from build123d import *

# Parameters (mm, degrees)
SKETCH1_W                      = 200
SKETCH1_H                      = 120
BOSS_EXTRUDE1_DEPTH            = 100
SHELL1_T                       = -3
CUT_EXTRUDE1_REACH             = 233.517
SKETCH5_W                      = 10
SKETCH5_H                      = 10
CUT_EXTRUDE1_DIRECTION_2_DEPTH = 232.516738056
FILLET2_R                      = 10
FILLET3_R                      = 10


with BuildPart() as part:
    # Sketch1 → Boss-Extrude1 (new body)
    with BuildSketch(Plane(origin=(0, 0, 0), x_dir=(1, 0, 0), z_dir=(0, 1, 0))):
        Rectangle(SKETCH1_W, SKETCH1_H)
    extrude(amount=BOSS_EXTRUDE1_DEPTH)

    # Shell1
    shell1_openings = [part.faces().sort_by_distance(p)[0] for p in [
        (0, 100, 0),
    ]]
    offset(amount=SHELL1_T, openings=shell1_openings, kind=Kind.INTERSECTION)

    # Sketch5 → Cut-Extrude1 (cut, up to next)
    with BuildSketch(Plane(origin=(100, 0, 0), x_dir=(0, 0, -1), z_dir=(1, 0, 0)), mode=Mode.PRIVATE) as cut_extrude1_sk1:
        with Locations((-50, 10)):
            Rectangle(SKETCH5_W, SKETCH5_H)
    cut_extrude1_tool1 = extrude(cut_extrude1_sk1.sketch, amount=-CUT_EXTRUDE1_REACH, mode=Mode.PRIVATE) & part.part
    add(cut_extrude1_tool1.solids().sort_by_distance((100, 10, 50))[0], mode=Mode.SUBTRACT)

    # Sketch5 → Cut-Extrude1 direction 2 (cut)
    with BuildSketch(Plane(origin=(100, 0, 0), x_dir=(0, 0, -1), z_dir=(1, 0, 0))):
        with Locations((-50, 10)):
            Rectangle(SKETCH5_W, SKETCH5_H)
    extrude(amount=CUT_EXTRUDE1_DIRECTION_2_DEPTH, mode=Mode.SUBTRACT)

    # Fillet2
    # the kernel refuses this fillet: 10 mm, written as the material it takes off along each edge
    with BuildSketch(Plane(origin=(-100, -25, -60), x_dir=(1, 0, 0), z_dir=(0, 1, 0)), Plane(origin=(-100, -25, 60), x_dir=(0, 0, -1), z_dir=(0, 1, 0))) as fillet2_piece_1:
        with BuildLine():
            CenterArc((FILLET2_R, -FILLET2_R), FILLET2_R, 90, 90)
            Line((0, -FILLET2_R), (0, 0))
            Line((0, 0), (FILLET2_R, 0))
        make_face()
    extrude(amount=150, mode=Mode.SUBTRACT)
    with BuildSketch(Plane(origin=(100, -25, 60), x_dir=(0, 0, -1), z_dir=(0, 1, 0)), Plane(origin=(100, -25, -60), x_dir=(-1, 0, 0), z_dir=(0, 1, 0))) as fillet2_piece_2:
        with BuildLine():
            CenterArc((FILLET2_R, FILLET2_R), FILLET2_R, 180, 90)
            Line((0, FILLET2_R), (0, 0))
            Line((0, 0), (FILLET2_R, 0))
        make_face()
    extrude(amount=150, mode=Mode.SUBTRACT)

    # Fillet3
    # the kernel refuses this fillet: 10 mm, written as the material it adds along each edge
    with BuildSketch(Plane(origin=(-97, 100, 57), x_dir=(0, 0, -1), z_dir=(0, -1, 0))) as fillet3_piece_1:
        with BuildLine():
            CenterArc((FILLET3_R, FILLET3_R), FILLET3_R, 180, 90)
            Line((0, FILLET3_R), (0, 0))
            Line((0, 0), (FILLET3_R, 0))
        make_face()
    extrude(amount=97)
    with BuildSketch(Plane(origin=(97, 100, 57), x_dir=(0, 0, -1), z_dir=(0, -1, 0))) as fillet3_piece_2_section:
        with BuildLine():
            CenterArc((FILLET3_R, -FILLET3_R), FILLET3_R, 90, 90)
            Line((0, -FILLET3_R), (0, 0))
            Line((0, 0), (FILLET3_R, 0))
        make_face()
    fillet3_piece_2 = extrude(amount=97, mode=Mode.PRIVATE)
    fillet3_piece_2 = split(fillet3_piece_2, bisect_by=Plane(origin=(96.033482281, 15, 52.791302356), z_dir=(0, 1, 0)), keep=Keep.TOP, mode=Mode.PRIVATE)
    fillet3_piece_2 = split(fillet3_piece_2, bisect_by=Plane(origin=(96.033482281, 57.5, 55), z_dir=(0, 0, -1)), keep=Keep.TOP, mode=Mode.PRIVATE)
    add(fillet3_piece_2)
    with BuildSketch(Plane(origin=(97, 100, 57), x_dir=(0, 0, -1), z_dir=(0, -1, 0))) as fillet3_piece_3_section:
        with BuildLine():
            CenterArc((FILLET3_R, -FILLET3_R), FILLET3_R, 90, 90)
            Line((0, -FILLET3_R), (0, 0))
            Line((0, 0), (FILLET3_R, 0))
        make_face()
    fillet3_piece_3 = extrude(amount=97, mode=Mode.PRIVATE)
    fillet3_piece_3 = split(fillet3_piece_3, bisect_by=Plane(origin=(93.714174943, 15, 56.26775421), z_dir=(0, 1, 0)), keep=Keep.TOP, mode=Mode.PRIVATE)
    fillet3_piece_3 = split(fillet3_piece_3, bisect_by=Plane(origin=(93.714174943, 57.5, 55), z_dir=(0, 0, 1)), keep=Keep.TOP, mode=Mode.PRIVATE)
    add(fillet3_piece_3)
    with BuildSketch(Plane(origin=(97, 100, 57), x_dir=(0, 0, -1), z_dir=(0, -1, 0))) as fillet3_piece_4_section:
        with BuildLine():
            CenterArc((FILLET3_R, -FILLET3_R), FILLET3_R, 90, 90)
            Line((0, -FILLET3_R), (0, 0))
            Line((0, 0), (FILLET3_R, 0))
        make_face()
    fillet3_piece_4 = extrude(amount=97, mode=Mode.PRIVATE)
    fillet3_piece_4 = split(fillet3_piece_4, bisect_by=Plane(origin=(93.714174943, 15, 56.26775421), z_dir=(0, -1, 0)), keep=Keep.TOP, mode=Mode.PRIVATE)
    fillet3_piece_4 = split(fillet3_piece_4, bisect_by=Plane(origin=(93.714174943, 10, 55), z_dir=(0, 0, 1)), keep=Keep.TOP, mode=Mode.PRIVATE)
    fillet3_piece_4 = split(fillet3_piece_4, bisect_by=Plane(origin=(93.714174943, 5, 56.26775421), z_dir=(0, 1, 0)), keep=Keep.TOP, mode=Mode.PRIVATE)
    add(fillet3_piece_4)
    with BuildSketch(Plane(origin=(97, 100, 57), x_dir=(0, 0, -1), z_dir=(0, -1, 0))) as fillet3_piece_5_section:
        with BuildLine():
            CenterArc((FILLET3_R, -FILLET3_R), FILLET3_R, 90, 90)
            Line((0, -FILLET3_R), (0, 0))
            Line((0, 0), (FILLET3_R, 0))
        make_face()
    fillet3_piece_5 = extrude(amount=97, mode=Mode.PRIVATE)
    fillet3_piece_5 = split(fillet3_piece_5, bisect_by=Plane(origin=(96.033482281, 4, 55), z_dir=(0, 0, -1)), keep=Keep.TOP, mode=Mode.PRIVATE)
    fillet3_piece_5 = split(fillet3_piece_5, bisect_by=Plane(origin=(96.033482281, 5, 52.791302356), z_dir=(0, -1, 0)), keep=Keep.TOP, mode=Mode.PRIVATE)
    add(fillet3_piece_5)
    with BuildSketch(Plane(origin=(97, 100, 57), x_dir=(0, 0, -1), z_dir=(0, -1, 0))) as fillet3_piece_6_section:
        with BuildLine():
            CenterArc((FILLET3_R, -FILLET3_R), FILLET3_R, 90, 90)
            Line((0, -FILLET3_R), (0, 0))
            Line((0, 0), (FILLET3_R, 0))
        make_face()
    fillet3_piece_6 = extrude(amount=97, mode=Mode.PRIVATE)
    fillet3_piece_6 = split(fillet3_piece_6, bisect_by=Plane(origin=(93.714174943, 4, 55), z_dir=(0, 0, 1)), keep=Keep.TOP, mode=Mode.PRIVATE)
    fillet3_piece_6 = split(fillet3_piece_6, bisect_by=Plane(origin=(93.714174943, 5, 56.26775421), z_dir=(0, -1, 0)), keep=Keep.TOP, mode=Mode.PRIVATE)
    add(fillet3_piece_6)
    with BuildSketch(Plane(origin=(-97, 3, -57), x_dir=(1, 0, 0), z_dir=(0, 1, 0)), Plane(origin=(97, 100, -57), x_dir=(-1, 0, 0), z_dir=(0, -1, 0))) as fillet3_piece_7:
        with BuildLine():
            CenterArc((FILLET3_R, -FILLET3_R), FILLET3_R, 90, 90)
            Line((0, -FILLET3_R), (0, 0))
            Line((0, 0), (FILLET3_R, 0))
        make_face()
    extrude(amount=97)


solid = part.part
Can you work these out from the model? Positions are in its coordinate system, mm. A direction names the side the tool comes from. Give positions to 0.01 mm unless a question says otherwise; leave off trailing zeros. Order: outer loops, then holes, each group sorted by start corner. A loop starts at its lowest first (then second) coordinate and runs counter-clockwise, first axis right, second up. Notation, with made-up numbers: (48, 45.25) - (65, 45.25) arc R13 ccw to (65, 55.25) - close; hole circle Ø1 at (21.5, -19). An arc over 180 degrees is marked (long way). Write each question's results on one line, items separated by ' | '.
1) Suppose I cut it at B-B, the plane x = 25.5. Write out the boundary of the cut face in (y, z).
Final values:
outline: (0, -60) - (100, -60) - (100, -57) - (3, -57) - (3, 57) - (100, 57) - (100, 60) - (0, 60) - close
2) If we mould it in two halves opening along X, with no side actions, what happens to faces 1 (the face through (-1, 51, -57)), 2 (the face through (97.15, 49.3, -56.99)), 3 (the face through (-97.15, 49.3, 56.99)), 4 (the face through (96, 10, 55))? For each: pulls with the +X half, pulls with the -X half, needs draft (parallel to the pull), parting line crosses it, or undercut.
Final values:
face 1: undercut | face 2: pulls with the +X half | face 3: pulls with the -X half | face 4: needs draft
3) On a 3-axis mill with a long thin cutter (end or side, diameter ignored), from which of +Z, -Z, +X, -X, +Y, -Y can I reach the whole of each face in a straight line? I mean faces 5 (the face through (93.99, 52.18, -54.15)), 6 (the face through (-96.99, 49.3, -57.15)), 7 (the face through (98, 5, 51)). Say none if no direction works.
Final values:
face 5: +Y | face 6: -Z, -X, +Y, -Y | face 7: +X
4) Suppose I cut it at A-A, the plane y = 58. Write out the boundary of the cut face in (x, z).
Final values:
outline: (-100, -50) arc R10 ccw to (-90, -60) - (90, -60) arc R10 ccw to (100, -50) - (100, 50) arc R10 ccw to (90, 60) - (-90, 60) arc R10 ccw to (-100, 50) - close; hole (-97, -47) arc R10 ccw to (-87, -57) - (87, -57) arc R10 ccw to (97, -47) - (97, 47) arc R10 ccw to (87, 57) - (-87, 57) arc R10 ccw to (-97, 47) - close
5) I'm going to push flat-ended pins straight in: pin 1 Ø3.5 at (x, y) = (99, 11) entering from +Z; pin 2 Ø7.5 at (x, z) = (95, 49.5) entering from -Y; pin 3 Ø3 at (x, y) = (96.5, 10) entering from -Z; pin 4 Ø1 at (x, z) = (16.5, -21) entering from +Y. Where does each tip first touch, or does it pass through?
Final values:
pin 1: stops at z = 56.89 | pin 2: stops at y = 0 | pin 3: stops at z = -58.66 | pin 4: stops at y = 3
6) Suppose I cut it at C-C, the plane z = -31. Write out the boundary of the cut face in (x, y), then the cut area to 3 significant figures.
Final values:
outline: (-100, 0) - (100, 0) - (100, 100) - (97, 100) - (97, 3) - (-97, 3) - (-97, 100) - (-100, 100) - close | area: 1,180 mm^2
7) Please list where these lines run through material, in increasing order: line 1 along X through (y, z) = (73.5, -18); line 2 along Z through (x, y) = (-29.5, 41.5); line 3 along Y through (x, z) = (-35, -7). Write a range as [from, to].
Final values:
line 1: x = [-100, -97], [97, 100] | line 2: z = [-60, -57], [57, 60] | line 3: y = [0, 3]
